Work out the finished part from the listing and answer in its coordinate system (mm). A direction names the side the tool comes from. Coordinates: 2 decimals unless noted, no trailing zeros. Order: outer loops, then holes, each group sorted by start corner. A loop starts at its lowest first (then second) coordinate and runs counter-clockwise, first axis right, second up. Notation, with made-up numbers: (10, -6) -> (19, -6) arc R3 ccw to (19, -1) -> close; hole circle Ø1 at (70.25, 4). An arc over 180 degrees is marked (long way). Write item = value, one per line. Start each with the question number.
Q1. The part is cut by section B-B, the plane x = 60. Determine the outline of the cut face in (y, z).
Q2. The part is cut by section C-C, the plane y = 1.95. Determine the outline of the cut face in (x, z).
Q3. Flat-ended cylindrical pins translate along their axes: pin 1 (6 mm diameter, centred on x = -70, z = 0, fed in from +Y); pin 2 (1.5 mm diameter, centred on x = 20, y = 4.5, fed in from +Z); pin 3 (0.9 mm diameter, centred on y = 5, z = 0, fed in from +X). Find the tip coordinate at first contact, or state that the pin passes through.
Q4. The part is cut by section D-D, the plane x = 27.5. Determine the outline of the cut face in (y, z).
Q5. Straight lines are drawn through the part: L1, parallel to X at y = 0.5, z = -2; L2, parallel to X at y = 1.85, z = 1.75; L3, parallel to Z at x = -70, y = 1. For each, find the intervals that lie inside material, in ascending order. Write a range as from..to.
Q6. Which of the six approach directions +Z, -Z, +X, -X, +Y, -Y give full straight-line access (tool end or side, diameter ignored) to faces 1 (the flat face through (-1, 4, -1.5)), 2 (the flat face through (1, 4, 1.5)), 3 (the flat face through (50, 4, 0)), 4 (the flat face through (75, 1, 0)), 5 (the flat face through (-50, 4, 0))?
Q7. The part is cut by section A-A, the plane z = 0. Determine the outline of the cut face in (x, y).
Autodesk Inventor part; units mm, degrees
ref_plane "YZ Plane" through (0, 0, 0) normal (1, 0, 0) x (0, 1, 0)
ref_plane "XZ Plane" through (0, 0, 0) normal (0, 1, 0) x (-1, 0, 0)
ref_plane "XY Plane" through (0, 0, 0) normal (0, 0, 1) x (1, 0, 0)
sketch "Sketch1" plane through (0, 0, 0) normal (0, 1, 0) x (-1, 0, 0)
  line L0 (-75, 9) -> (0, 9)
  line L1 (75, 9) -> (75, -9)
  line L2 (75, -9) -> (0, -9)
  line L3 (-75, -9) -> (-75, 9)
  line L4 (-75, 0) -> (75, 0) construction
  circle A0 centre (-70, 0) radius 2.25
  circle A1 centre (-60, 0) radius 2.25
  line L5 (0, 9) -> (75, 9)
  line L6 (0, -9) -> (-75, -9)
  line L7 (-55, 9) -> (-55, -9)
  line L8 (0, 37.7423) -> (0, -37.3462) construction
  circle A2 centre (70, 0) radius 2.25
  circle A3 centre (60, 0) radius 2.25
  line L9 (55, 9) -> (55, -9)
  point P0 (0, 0)
  dimension "d1" = 18
  dimension "d2" = 4.5
  dimension "d3" = 4.5
  dimension "d4" = 5
  dimension "d5" = 15
  dimension "d17" = 5
  dimension "d18" = 110
  dimension "d19" = 5
extrude "Extrusion1" add sketch "Sketch1" along normal blind 3
sketch "Sketch2" plane through (0, 3, 0) normal (0, 1, 0) x (1, 0, 0)
  line L0 (-50, 1.5) -> (50, 1.5)
  line L1 (50, 1.5) -> (50, -1.5)
  line L2 (50, -1.5) -> (-50, -1.5)
  line L3 (-50, -1.5) -> (-50, 1.5)
  point P0 (0, 0)
  point P1 (50, 0)
  point P2 (0, 1.5)
  dimension "d20" = 100
  dimension "d21" = 3
extrude "Extrusion3" add sketch "Sketch2" along normal blind 3
properties part number "TopSliderBar"
Model answer:
q1.outline = (0, -9) -> (3, -9) -> (3, -2.25) -> (0, -2.25) -> close; (0, 2.25) -> (3, 2.25) -> (3, 9) -> (0, 9) -> close
q2.outline = (-75, -9) -> (75, -9) -> (75, 9) -> (-75, 9) -> close; hole circle Ø4.5 at (-70, 0); hole circle Ø4.5 at (-60, 0); hole circle Ø4.5 at (60, 0); hole circle Ø4.5 at (70, 0)
q3.pin_1 = 3
q3.pin_2 = 1.5
q3.pin_3 = 50
q4.outline = (0, -9) -> (3, -9) -> (3, -1.5) -> (6, -1.5) -> (6, 1.5) -> (3, 1.5) -> (3, 9) -> (0, 9) -> close
q5.L1 = -75..-71.03, -68.97..-61.03, -58.97..58.97, 61.03..68.97, 71.03..75
q5.L2 = -75..-71.41, -68.59..-61.41, -58.59..58.59, 61.41..68.59, 71.41..75
q5.L3 = -9..-2.25, 2.25..9
q6.face_1 = -Z, +X, -X, +Y
q6.face_2 = +Z, +X, -X, +Y
q6.face_3 = +Z, -Z, +X, +Y
q6.face_4 = +Z, -Z, +X, +Y, -Y
q6.face_5 = +Z, -Z, -X, +Y
q7.outline = (-75, 0) -> (-72.25, 0) -> (-72.25, 3) -> (-75, 3) -> close; (-67.75, 0) -> (-62.25, 0) -> (-62.25, 3) -> (-67.75, 3) -> close; (-57.75, 0) -> (57.75, 0) -> (57.75, 3) -> (50, 3) -> (50, 6) -> (-50, 6) -> (-50, 3) -> (-57.75, 3) -> close; (62.25, 0) -> (67.75, 0) -> (67.75, 3) -> (62.25, 3) -> close; (72.25, 0) -> (75, 0) -> (75, 3) -> (72.25, 3) -> close
